```python
from build123d import *

# Parameters (mm, degrees)
SKETCH1_W                      = 50
SKETCH1_H                      = 25
BOSS_EXTRUDE1_DEPTH            = 5
SKETCH2_W                      = 10
SKETCH2_H                      = 50
BOSS_EXTRUDE2_DEPTH            = 3.5
SKETCH3_W                      = 10
SKETCH3_H                      = 4.126638733
BOSS_EXTRUDE3_DEPTH            = 26.5
SKETCH4_W                      = 4.126638733
SKETCH4_H                      = 14
BOSS_EXTRUDE4_DEPTH            = 12.5
SKETCH5_W                      = 4.126638733
SKETCH5_H                      = 14
BOSS_EXTRUDE5_DEPTH            = 12.5
F_4_0_4_DIAMETER_HOLE1_D       = 4
F_4_0_4_DIAMETER_HOLE1_DEPTH   = 50
F_16_0_16_DIAMETER_HOLE1_D     = 16
F_16_0_16_DIAMETER_HOLE1_DEPTH = 5
FILLET1_R                      = 3


with BuildPart() as part:
    # Sketch1 → Boss-Extrude1 (new body)
    with BuildSketch(Plane.XZ.offset(5)):
        Rectangle(SKETCH1_W, SKETCH1_H)
    extrude(amount=-BOSS_EXTRUDE1_DEPTH)

    # Sketch2 → Boss-Extrude2 (add)
    with BuildSketch(Plane(origin=(0, 0, 0), x_dir=(-1, 0, 0), z_dir=(0, 1, 0))):
        with Locations((0, -12.5)):
            Rectangle(SKETCH2_W, SKETCH2_H)
    extrude(amount=BOSS_EXTRUDE2_DEPTH)

    # Sketch3 → Boss-Extrude3 (add)
    with BuildSketch(Plane.XZ):
        with Locations((0, -35.436680634)):
            Rectangle(SKETCH3_W, SKETCH3_H)
    extrude(amount=BOSS_EXTRUDE3_DEPTH)

    # Sketch4 → Boss-Extrude4 (add)
    with BuildSketch(Plane(origin=(5, 0, 0), x_dir=(0, 0, -1), z_dir=(1, 0, 0))):
        with Locations((35.436680634, -19.5)):
            Rectangle(SKETCH4_W, SKETCH4_H)
    extrude(amount=BOSS_EXTRUDE4_DEPTH)

    # Sketch5 → Boss-Extrude5 (add)
    with BuildSketch(Plane.ZY.offset(5)):
        with Locations((-35.436680634, -19.5)):
            Rectangle(SKETCH5_W, SKETCH5_H)
    extrude(amount=BOSS_EXTRUDE5_DEPTH)

    # Ø4.0 (4) Diameter Hole1
    with Locations(Plane(origin=(0, 0, -37.5), x_dir=(-1, 0, 0), z_dir=(0, 0, -1))):
        with Locations((0, -19.5)):
            Hole(F_4_0_4_DIAMETER_HOLE1_D / 2, depth=F_4_0_4_DIAMETER_HOLE1_DEPTH)

    # Ø16.0 (16) Diameter Hole1
    with Locations(Plane.XZ.offset(5)):
        with Locations((-12.6, 0)):
            f_16_0_16_diameter_hole1 = Hole(F_16_0_16_DIAMETER_HOLE1_D / 2, depth=F_16_0_16_DIAMETER_HOLE1_DEPTH)

    # Fillet1
    fillet1_edges = [part.edges().sort_by_distance(p)[0] for p in [
        (0, 3.5, 12.5),
        (0, 3.5, -37.5),
        (0, 0, -33.373361267),
        (5, -12.5, -35.436680634),
        (-5, -12.5, -35.436680634),
        (25, -2.5, 12.5),
        (25, -2.5, -12.5),
        (-25, -2.5, -12.5),
        (-25, -2.5, 12.5),
    ]]
    fillet(fillet1_edges, radius=FILLET1_R)

    # Mirror1: Ø16.0 (16) Diameter Hole1 across plane
    add(f_16_0_16_diameter_hole1.mirror(Plane(origin=(0, 0, 0), x_dir=(0, 0, 1), z_dir=(1, 0, 0))), mode=Mode.SUBTRACT)


solid = part.part
```
CAD build for the part. Positions are in the model's coordinates, mm. A direction names the side the tool comes from. Coordinates: 2 decimals unless noted, no trailing zeros. Order: outer loops, then holes, each group sorted by start corner. A loop starts at its lowest first (then second) coordinate and runs counter-clockwise, first axis right, second up. Notation, with made-up numbers: (-13, 72.25) - (23, 72.25) arc R26 ccw to (23, 100.25) - close; hole circle Ø2 at (-18, 0.5). An arc over 180 degrees is marked (long way). Use a Markdown table: item, result. Add a question column.
(1) Saw through at A-A (y = -19.5). Give the cut face in (x, z).
(2) Which spindle directions (+Z, -Z, +X, -X, +Y, -Y) get a long thin tool onto all of the face, cutting with end or side? Do faces 1 (the face through (-13, -12.5, -35)), 2 (the face through (0, 0, -21)), 3 (the face through (-24.1, -2.46, 11.64)), 4 (the face through (0, -5, 0)). Say none if no direction does.
(3) Saw through at C-C (z = 0). Give the cut face in (x, y).
(4) Flat gauge pins, fed straight in: pin 1 (3.5 mm diameter, centred on x = -14, z = -34.5, fed in from +Y); pin 2 (5 mm diameter, centred on x = -5, z = 3, fed in from -Y); pin 3 (4.5 mm diameter, centred on x = 0, y = -19.5, fed in from +Z); pin 4 (6.5 mm diameter, centred on y = -1, z = -11.5, fed in from -X). Where does each tip first touch, or does it go through?
(5) Pull direction Z, two halves, no side cores. Call faces 5 (the face through (-0.07, 2.6, -36.64)), 6 (the face through (0.07, -0.902, -32.518)), 7 (the face through (5, 0.4, -16.3)), 8 (the face through (0, -3, -12.5)): +Z half, -Z half, draft (parallel to the pull), parting line (faces both ways), or undercut.
(6) Saw through at B-B (x = 12.6). Give the cut face in (y, z).
(7) Saw through at D-D (x = 0). Give the cut face in (y, z).
(8) Drill centre lines: line 1 along X through (y, z) = (-3.35, 0); line 2 along Z through (x, y) = (12.6, -2.45); line 3 along Y through (x, z) = (-20.5, -10.5). Where is each one in solid material? Low to high. Write a range as [from, to].
Solved:
| question | item | result |
|---|---|---|
| 1 | outline | (-17.5, -37.5) - (-2, -37.5) - (-2, -33.37) - (-17.5, -33.37) - close; (2, -37.5) - (17.5, -37.5) - (17.5, -33.37) - (2, -33.37) - close |
| 2 | face 1 | +Z, -Z, -X, +Y |
| 2 | face 2 | +X, -X, -Y |
| 2 | face 3 | +Z, -X, +Y, -Y |
| 2 | face 4 | +Z, +X, -X, -Y |
| 3 | outline | (-25, -5) - (-20.6, -5) - (-20.6, 0) - (-25, 0) - close; (-5, 0) - (-4.6, 0) - (-4.6, -5) - (4.6, -5) - (4.6, 0) - (5, 0) - (5, 3.5) - (-5, 3.5) - close; (20.6, -5) - (25, -5) - (25, 0) - (20.6, 0) - close |
| 4 | pin 1 | stops at y = -12.5 |
| 4 | pin 2 | stops at y = -5 |
| 4 | pin 3 | stops at z = -33.37 |
| 4 | pin 4 | stops at x = -25 |
| 5 | face 5 | -Z half |
| 5 | face 6 | undercut |
| 5 | face 7 | draft |
| 5 | face 8 | undercut |
| 6 | outline | (-26.5, -37.5) - (-12.5, -37.5) - (-12.5, -33.37) - (-26.5, -33.37) - close; (-5, -12.5) - (0, -12.5) - (0, -8) - (-5, -8) - close; (-5, 8) - (0, 8) - (0, 12.5) - (-5, 12.5) - close |
| 7 | outline | (-26.5, -37.5) - (-21.5, -37.5) - (-21.5, -33.37) - (-26.5, -33.37) - close; (-17.5, -37.5) - (0.5, -37.5) arc R3 ccw to (3.5, -34.5) - (3.5, 9.5) arc R3 ccw to (0.5, 12.5) - (-5, 12.5) - (-5, -12.5) - (0, -12.5) - (0, -30.37) arc R3 cw to (-3, -33.37) - (-17.5, -33.37) - close |
| 8 | line 1 | x = [-25, -20.6], [-4.6, 4.6], [20.6, 25] |
| 8 | line 2 | z = [-12.5, -8], [8, 12.5] |
| 8 | line 3 | y = [-5, 0] |
